Geometry check sheet. Reference: drawing and pictorial views, mm from the part's lowest x, y, z. A direction names the side the tool comes from. Round coordinates to 2 decimals unless told otherwise and drop trailing zeros. Write each loop counter-clockwise with the first axis right and the second up, starting at its lowest first coordinate (ties: lowest second). Pieces come first, ordered by that corner, then holes. Notation, with made-up numbers: (80, -29) -> (110, -29) arc R26 cw to (110, 0) -> close; hole circle Ø6 at (75.5, -18). An arc over 180 degrees is marked (long way). Write item = value, one per line.
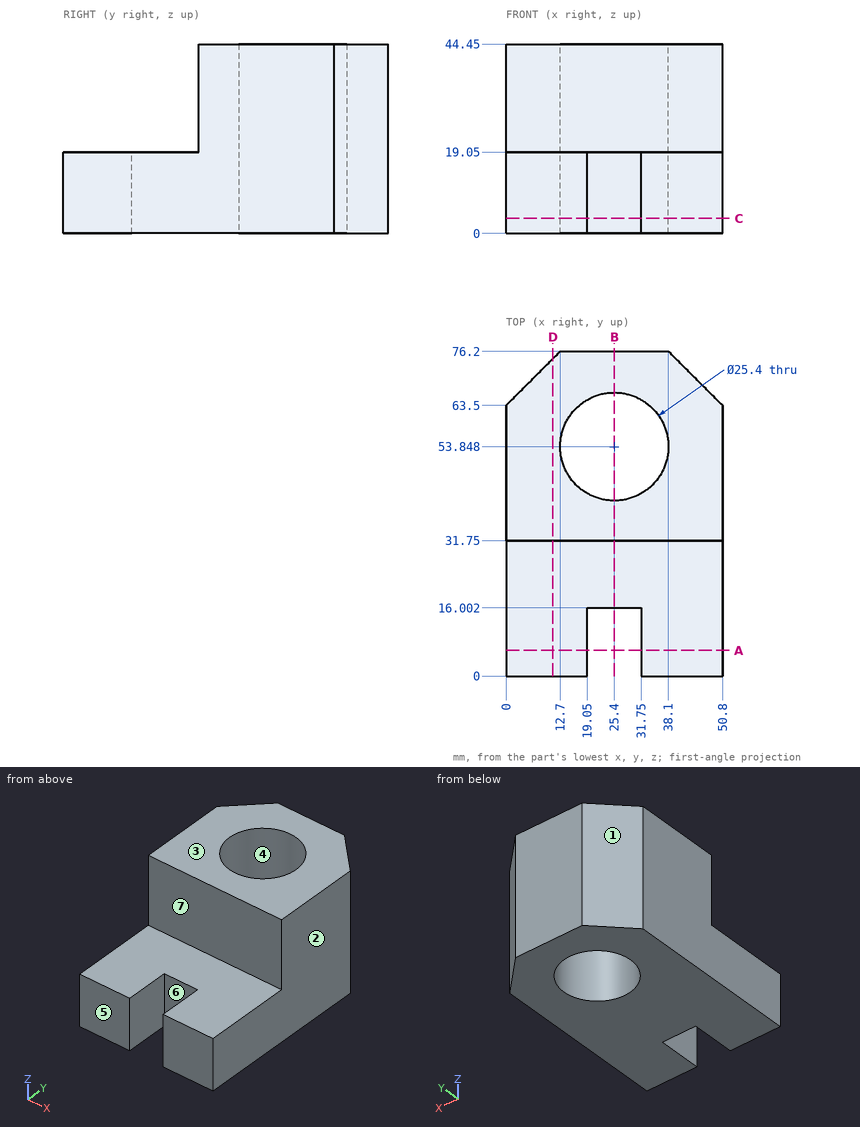
(1) Sectioned sample at D-D on x = 11. Enter the section's corners in (y, z).
Worked answers:
outline = (0, 0) -> (74.5, 0) -> (74.5, 44.45) -> (31.75, 44.45) -> (31.75, 19.05) -> (0, 19.05) -> close
(2) Access from +Z, -Z, +X, -X, +Y, -Y to the whole of each face (thin tool, end or side, straight path). Record for the marked faces 5, 6 and 7.
Worked answers:
face_5 = +Z, -Z, +X, -X, -Y
face_6 = +Z, -Z, -Y
face_7 = +Z, +X, -X, -Y
(3) Sectioned sample at B-B on x = 25.4. Enter the section's corners in (y, z).
Worked answers:
outline = (16, 0) -> (41.15, 0) -> (41.15, 44.45) -> (31.75, 44.45) -> (31.75, 19.05) -> (16, 19.05) -> close; (66.55, 0) -> (76.2, 0) -> (76.2, 44.45) -> (66.55, 44.45) -> close
(4) Go/stop test with flat-tipped pins: P1, Ø6.5, axis at x = 25.5, z = 12, coming from the -Y side; P2, Ø15, axis at x = 25.4, y = 53.848, coming from the +Z side; P3, Ø8, axis at x = 8.5, z = 37.5, coming from the +Y side; P4, Ø4, axis at x = 28.5, z = 22, coming from the -Y side. Record where each tip stops, or that it passes through.
Worked answers:
P1 = 16
P2 = through
P3 = 76
P4 = 31.75
(5) Sectioned sample at A-A on y = 6. Enter the section's corners in (x, z), then the cut area to 3 significant figures.
Worked answers:
outline = (0, 0) -> (19.05, 0) -> (19.05, 19.05) -> (0, 19.05) -> close; (31.75, 0) -> (50.8, 0) -> (50.8, 19.05) -> (31.75, 19.05) -> close
area = 726 mm²
(6) Sectioned sample at C-C on z = 3.5. Enter the section's corners in (x, y).
Worked answers:
outline = (0, 0) -> (19.05, 0) -> (19.05, 16) -> (31.75, 16) -> (31.75, 0) -> (50.8, 0) -> (50.8, 63.5) -> (38.1, 76.2) -> (12.7, 76.2) -> (0, 63.5) -> close; hole circle Ø25.4 at (25.4, 53.85)
(7) Material ranges on L1, parallel to Y at x = 25.4, z = 35; L2, parallel to Y at x = 25.4, z = 14.5; L3, parallel to Z at x = 6, y = 25, recorded low to high. Write a range as [from, to].
Worked answers:
L1 = [31.75, 41.15], [66.55, 76.2]
L2 = [16, 41.15], [66.55, 76.2]
L3 = [0, 19.05]
(8) Release check for a two-part mould opening along X. For the marked faces 1, 2, 3 and 4 record: pulls with the +X half, pulls with the -X half, needs draft (parallel to the pull), parting line crosses it, or undercut.
Worked answers:
face_1 = pulls with the -X half
face_2 = pulls with the +X half
face_3 = needs draft
face_4 = undercut
